Build history of the part. All positions in model axes, mm. A direction names the side the tool comes from. Round coordinates to 2 decimals unless told otherwise and drop trailing zeros. Loops run counter-clockwise (first coordinate to the right, second up) from the corner with the lowest first, then second, coordinate; pieces in that order, holes last. Notation, with made-up numbers: (13, 70.25) - (25, 70.25) arc R18 cw to (25, 83.25) - close; hole circle Ø10 at (33.25, 6.5). An arc over 180 degrees is marked (long way). Answer as CSV lines item,"result". Start each with the question number.
```python
from build123d import *

# Parameters (mm, degrees)
SKETCH1_R           = 2.4892
BOSS_EXTRUDE1_DEPTH = 2.286


with BuildPart() as part:
    # Sketch1 → Boss-Extrude1 (new body)
    with BuildSketch(Plane(origin=(0, 0, 0), x_dir=(-1, 0, 0), z_dir=(0, 0, -1))):
        Polygon((12.7, 12.7), (-50.8, 12.7), (-50.8, -12.7), (-12.7, -12.7), (-12.7, -50.8), (12.7, -50.8), align=None)
        with Locations((0, -25.4)):
            Circle(SKETCH1_R, mode=Mode.SUBTRACT)
        with Locations((-38.1, 0)):
            Circle(SKETCH1_R, mode=Mode.SUBTRACT)
        with Locations((-12.7, 0)):
            Circle(SKETCH1_R, mode=Mode.SUBTRACT)
        Circle(SKETCH1_R, mode=Mode.SUBTRACT)
        with Locations((-25.4, 0)):
            Circle(SKETCH1_R, mode=Mode.SUBTRACT)
        with Locations((0, -12.7)):
            Circle(SKETCH1_R, mode=Mode.SUBTRACT)
        with Locations((0, -38.1)):
            Circle(SKETCH1_R, mode=Mode.SUBTRACT)
    extrude(amount=-BOSS_EXTRUDE1_DEPTH)


solid = part.part
```
Q1. Pin check, flat tip, straight feed: pin 1 Ø1.1 at (y, z) = (-26.5, 1.5) entering from +X. Stop position of the tip, or through.
Q2. Band-saw the part on C-C, the plane x = 38.1. List the corners of the cut face in (y, z), then the cut area to 3 significant figures.
Q3. Tool access for faces 4 (the flat face through (-12.7, -19, 1)), 5 (the flat face through (12.7, -31, 1)): list every direction of +Z, -Z, +X, -X, +Y, -Y with a clear straight run to the whole face (end or side of a thin tool).
Q4. Band-saw the part on B-B, the plane z = 0.85. List the corners of the cut face in (x, y), then the cut area to 3 significant figures.
Q5. Two-plate mould, pull along X, no slides. Class faces 1 (the cylindrical face through (0.54, -27.83, 1.13)), 2 (the flat face through (19, 12.7, 1)), 3 (the flat face through (50.8, 0, 1)): released by +X, released by -X, zero draft, split by the parting line, or undercut.
Q6. Band-saw the part on A-A, the plane y = 0. List the corners of the cut face in (x, z), then the cut area to 3 significant figures.
Q7. Wall check: probe 1 along Y at (x, z) = (0, 0.9); probe 2 along Y at (x, z) = (25.4, 0.5); probe 3 along Y at (x, z) = (33.5, 0.7). Give the ranges that are in metal, low to high. Write a range as [from, to].
Reported:
1,pin 1,"stops at x = 12.7"
2,outline,"(-12.7, 0) - (-2.49, 0) - (-2.49, 2.29) - (-12.7, 2.29) - close; (2.49, 0) - (12.7, 0) - (12.7, 2.29) - (2.49, 2.29) - close"
2,area,"46.7 mm2"
3,face 4,"+Z, -Z, -X, +Y, -Y"
3,face 5,"+Z, -Z, +X, -Y"
4,outline,"(-12.7, -50.8) - (12.7, -50.8) - (12.7, -12.7) - (50.8, -12.7) - (50.8, 12.7) - (-12.7, 12.7) - close; hole circle Ø4.98 at (0, -38.1); hole circle Ø4.98 at (0, -25.4); hole circle Ø4.98 at (0, -12.7); hole circle Ø4.98 at (0, 0); hole circle Ø4.98 at (12.7, 0); hole circle Ø4.98 at (25.4, 0); hole circle Ø4.98 at (38.1, 0)"
4,area,"2,440 mm2"
5,face 1,"undercut"
5,face 2,"zero draft"
5,face 3,"released by +X"
6,outline,"(-12.7, 0) - (-2.49, 0) - (-2.49, 2.29) - (-12.7, 2.29) - close; (2.49, 0) - (10.21, 0) - (10.21, 2.29) - (2.49, 2.29) - close; (15.19, 0) - (22.91, 0) - (22.91, 2.29) - (15.19, 2.29) - close; (27.89, 0) - (35.61, 0) - (35.61, 2.29) - (27.89, 2.29) - close; (40.59, 0) - (50.8, 0) - (50.8, 2.29) - (40.59, 2.29) - close"
6,area,"99.6 mm2"
7,probe 1,"y = [-50.8, -40.59], [-35.61, -27.89], [-22.91, -15.19], [-10.21, -2.49], [2.49, 12.7]"
7,probe 2,"y = [-12.7, -2.49], [2.49, 12.7]"
7,probe 3,"y = [-12.7, 12.7]"
